CAD build for the part. Positions are in the model's coordinates, mm. Coordinates: 2 decimals unless noted, no trailing zeros. Loops run counter-clockwise (first coordinate to the right, second up) from the corner with the lowest first, then second, coordinate; pieces in that order, holes last.
1) Saw through at A-A, the plane x = -12.7. Write the cut outline in (y, z), and give its area (3 significant figures).
2) Saw through at B-B, the plane z = 2. Write the cut outline in (x, y), and give its area (3 significant figures).
3) Saw through at D-D, the plane z = -5. Write the cut outline in (x, y), and give its area (3 significant figures).
4) Pin check, flat tips, straight feed: pin 1 Ø3 at (x, z) = (-35, -5) entering from -Y; pin 2 Ø1.5 at (y, z) = (2, -16) entering from +X; pin 3 Ø1.5 at (x, y) = (-39.5, 2) entering from -Z; pin 4 Ø1 at (y, z) = (1, -3) entering from -X. Stop position of each tip, or through.
5) Saw through at C-C, the plane y = 0.7. Write the cut outline in (x, z).
6) Wall check: line 1 along X through (y, z) = (1.3, 0); line 2 along Z through (x, y) = (-19.5, 1.55); line 3 along X through (y, z) = (1.75, -5.5). Give the ranges that are in metal, low to high.
```python
from build123d import *

# Parameters (mm, degrees)
BOSS_EXTRUDE1_DEPTH = 3
SKETCH2_R           = 8.15
CUT_EXTRUDE4_DEPTH  = 49.559242169
SKETCH3_R           = 2.5
CUT_EXTRUDE5_DEPTH  = 10
CUT_EXTRUDE6_DEPTH  = 10


with BuildPart() as part:
    # Sketch1 → Boss-Extrude1 (new body)
    with BuildSketch(Plane(origin=(0, 0, 0), x_dir=(1, 0, 0), z_dir=(0, 1, 0))):
        Polygon((-45, 15), (-30, 15), (-30, 18), (-15, 18), (-15, 15), (15, 15), (15, 18), (30, 18), (30, 15), (45, 15), (45, -15), (-45, -15), align=None)
    extrude(amount=BOSS_EXTRUDE1_DEPTH)

    # Sketch2 → Cut-Extrude4 (cut, through all)
    with BuildSketch(Plane(origin=(0, 0, 0), x_dir=(1, 0, 0), z_dir=(0, 1, 0))):
        with Locations(Location((-12.7, 0, 0), (0, 0, 270))):
            Circle(SKETCH2_R)
        with Locations(Location((12.7, 0, 0), (0, 0, 90))):
            Circle(SKETCH2_R)
    extrude(amount=CUT_EXTRUDE4_DEPTH, mode=Mode.SUBTRACT)

    # Sketch3 → Cut-Extrude5 (cut)
    with BuildSketch(Plane(origin=(0, 3, 0), x_dir=(1, 0, 0), z_dir=(0, 1, 0))):
        with Locations(Location((-35, 5, 0), (0, 0, 270))):
            Circle(SKETCH3_R)
    extrude(amount=-CUT_EXTRUDE5_DEPTH, mode=Mode.SUBTRACT)

    # Sketch4 → Cut-Extrude6 (cut)
    with BuildSketch(Plane(origin=(0, 3, 0), x_dir=(1, 0, 0), z_dir=(0, 1, 0))):
        with BuildLine():
            ThreePointArc((-23.786796564, -15), (-38.786796564, -8.786796564), (-45, 6.213203436))
            Line((-45, 6.213203436), (-45, -15))
            Line((-45, -15), (-23.786796564, -15))
        make_face()
        with BuildLine():
            ThreePointArc((45, 6.213203436), (38.786796564, -8.786796564), (23.786796564, -15))
            Line((23.786796564, -15), (45, -15))
            Line((45, -15), (45, 6.213203436))
        make_face()
    extrude(amount=-CUT_EXTRUDE6_DEPTH, mode=Mode.SUBTRACT)


solid = part.part
```
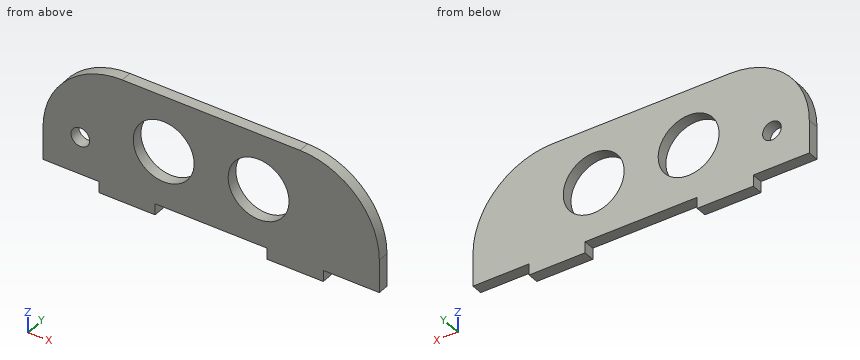
Data:
1. outline: (0, -15) - (3, -15) - (3, -8.15) - (0, -8.15) - close; (0, 8.15) - (3, 8.15) - (3, 15) - (0, 15) - close
1. area: 41.1 mm2
2. outline: (-43.35, 0) - (-20.6, 0) - (-20.6, 3) - (-43.35, 3) - close; (-4.8, 0) - (4.8, 0) - (4.8, 3) - (-4.8, 3) - close; (20.6, 0) - (43.35, 0) - (43.35, 3) - (20.6, 3) - close
2. area: 165 mm2
3. outline: (-44.97, 0) - (-37.5, 0) - (-37.5, 3) - (-44.97, 3) - close; (-32.5, 0) - (-19.14, 0) - (-19.14, 3) - (-32.5, 3) - close; (-6.26, 0) - (6.26, 0) - (6.26, 3) - (-6.26, 3) - close; (19.14, 0) - (44.97, 0) - (44.97, 3) - (19.14, 3) - close
3. area: 178 mm2
4. pin 1: passes through
4. pin 2: stops at x = 30
4. pin 3: stops at z = -15
4. pin 4: stops at x = -44.83
5. outline: (-45, -15) - (-30, -15) - (-30, -18) - (-15, -18) - (-15, -15) - (15, -15) - (15, -18) - (30, -18) - (30, -15) - (45, -15) - (45, -6.21) arc R21.21 ccw to (23.79, 15) - (-23.79, 15) arc R21.21 ccw to (-45, -6.21) - close; hole circle Ø5 at (-35, -5); hole circle Ø16.3 at (-12.7, 0); hole circle Ø16.3 at (12.7, 0)
6. line 1: x = -44.07 to -20.85, -4.55 to 4.55, 20.85 to 44.07
6. line 2: z = -18 to -4.49, 4.49 to 15
6. line 3: x = -44.99 to -37.45, -32.55 to -18.71, -6.69 to 6.69, 18.71 to 44.99
